from build123d import *

# Parameters (mm, degrees)
F1_DEPTH = 38.1
F2_R     = 5.08
F4_D     = 3.175


with BuildPart() as f1:
    # F0 (on Top) → F1 (new body)
    with BuildSketch(Plane.XY):
        with BuildLine():
            Line((32.319215, -2.299103), (32.319215, 1.700897))
            Line((32.319215, 1.700897), (36.015589, 1.700897))
            ThreePointArc((36.015589, 1.700897), (9.819215, 24.200897), (-16.377159, 1.700897))
            Line((-16.377159, 1.700897), (-12.680785, 1.700897))
            Line((-12.680785, 1.700897), (-12.680785, -2.299103))
            ThreePointArc((-12.680785, -2.299103), (9.819215, 20.200897), (32.319215, -2.299103))
        make_face()
        with BuildLine():
            Line((36.015589, 1.700897), (32.319215, 1.700897))
            Line((32.319215, 1.700897), (32.319215, -2.299103))
            Line((32.319215, -2.299103), (36.319215, -2.299103))
            ThreePointArc((36.319215, -2.299103), (36.2432, -0.293349), (36.015589, 1.700897))
        make_face()
        with BuildLine():
            Line((70.419215, 1.700897), (36.015589, 1.700897))
            ThreePointArc((36.015589, 1.700897), (36.2432, -0.293349), (36.319215, -2.299103))
            Line((36.319215, -2.299103), (70.419215, -2.299103))
            Line((70.419215, -2.299103), (70.419215, 1.700897))
        make_face()
        with BuildLine():
            Line((-12.680785, 1.700897), (-16.377159, 1.700897))
            ThreePointArc((-16.377159, 1.700897), (-16.604769, -0.293349), (-16.680785, -2.299103))
            Line((-16.680785, -2.299103), (-12.680785, -2.299103))
            Line((-12.680785, -2.299103), (-12.680785, 1.700897))
        make_face()
        with BuildLine():
            ThreePointArc((-16.680785, -2.299103), (-16.604769, -0.293349), (-16.377159, 1.700897))
            Line((-16.377159, 1.700897), (-50.780785, 1.700897))
            Line((-50.780785, 1.700897), (-50.780785, -2.299103))
            Line((-50.780785, -2.299103), (-16.680785, -2.299103))
        make_face()
    extrude(amount=F1_DEPTH)

    # F2
    f2_edges = [f1.edges().sort_by_distance(p)[0] for p in [
        (70.419215, -0.299103, 38.1),
        (70.419215, -0.299103, 0),
        (32.319215, -2.299103, 19.05),
        (-12.680785, -2.299103, 19.05),
        (-50.780785, -0.299103, 38.1),
        (-50.780785, -0.299103, 0),
        (-16.377159, 1.700897, 19.05),
        (36.015589, 1.700897, 19.05),
    ]]
    fillet(f2_edges, radius=F2_R)

    # F4 (through all)
    with Locations(Plane(origin=(0, 1.700897, 0), x_dir=(-1, 0, 0), z_dir=(0, 1, 0))):
        with Locations((-58.892906, 25.4), (-58.892906, 12.7), (38.062844, 12.7), (38.062844, 25.4)):
            Hole(F4_D / 2)


solid = f1.part
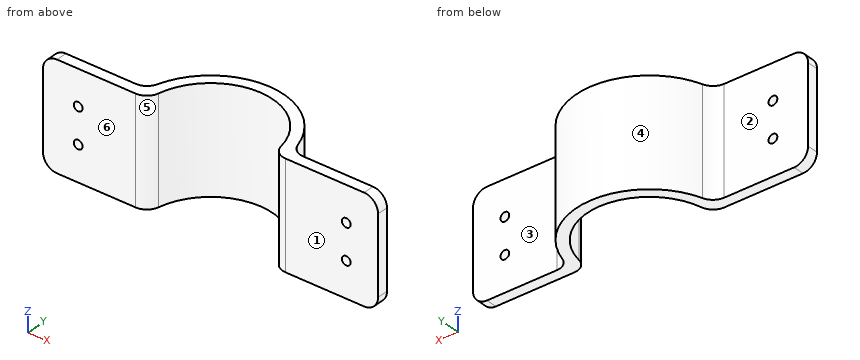
For this review, take the finished solid that the model builds, in its own axes (mm). Face numbers are marked on the shaded views. A direction names the side the tool comes from. Give positions to 0.01 mm unless a question says otherwise; leave off trailing zeros. Loops run counter-clockwise (first coordinate to the right, second up) from the corner with the lowest first, then second, coordinate; pieces in that order, holes last. Notation, with made-up numbers: M -2,39 L 51,39 A22 ccw 51,45 Z; hole C 22,85.5 d11. An arc over 180 degrees is marked long. Answer as a JSON object with one key per item and string values. Group by question number.
Q1. Add section B-B on z = 21. Give the boundary of the cut face in (x, y).
Q2. For probe 1 along Y at (x, z) = (41.5, 8.5); probe 2 along X at (y, z) = (16.5, 22.5); probe 3 along X at (y, z) = (15.5, 31), list the stretches that pass through material, from the lowest coordinate up. Write a range as [from, to].
Q3. Add section D-D on x = 19. Give the boundary of the cut face in (y, z).
Q4. Add section A-A on z = 12.7. Give the boundary of the cut face in (x, y).
Q5. Add section C-C on y = 11. Give the boundary of the cut face in (x, z).
Q6. Mouldability with a two-part tool opening along X and no side actions: class the marked faces 4, 5 and 6 as +X half, -X half, draft (parallel to the pull), parting line (faces both ways), or undercut.
Q7. Tool access review of the marked faces 1, 2 and 3: name each direction out of +Z, -Z, +X, -X, +Y, -Y from which nothing blocks a thin tool from reaching the whole face with its end or side.
Q8. Insertion check: P1, Ø15, axis at x = -40.5, z = 19, coming from the +Y side; P2, Ø12, axis at x = 39, y = 8, coming from the +Z side; P3, Ø8, axis at y = 11.5, z = 22.5, coming from the +X side; P4, Ø12, axis at y = 19.5, z = 16.5, coming from the +X side. Each pin has a flat end and moves straight along its axis. Give the tip position at first contact, or say it passes through.
Checked values:
{
 "1": {"outline": "M -50.78,-2.3 L -17.29,-2.3 A5.08 ccw -12.3,1.85 A22.5 cw 31.93,1.85 A5.08 ccw 36.93,-2.3 L 70.42,-2.3 L 70.42,1.7 L 40.07,1.7 A5.08 cw 35.2,5.32 A26.5 ccw -15.56,5.32 A5.08 cw -20.43,1.7 L -50.78,1.7 Z"},
 "2": {"probe 1": "[-2.3, 1.7]", "probe 2": "[-8.86, -2.54], [22.18, 28.5]", "probe 3": "[-9.81, -3.94], [23.58, 29.45]"},
 "3": {"outline": "M 18.24,0 L 22.56,0 L 22.56,38.1 L 18.24,38.1 Z"},
 "4": {"outline": "M -50.78,-2.3 L -39.65,-2.3 L -39.65,1.7 L -50.78,1.7 Z; M -36.48,-2.3 L -17.29,-2.3 A5.08 ccw -12.3,1.85 A22.5 cw 31.93,1.85 A5.08 ccw 36.93,-2.3 L 57.31,-2.3 L 57.31,1.7 L 40.07,1.7 A5.08 cw 35.2,5.32 A26.5 ccw -15.56,5.32 A5.08 cw -20.43,1.7 L -36.48,1.7 Z; M 60.48,-2.3 L 70.42,-2.3 L 70.42,1.7 L 60.48,1.7 Z"},
 "5": {"outline": "M -13.1,0 L -8.33,0 L -8.33,38.1 L -13.1,38.1 Z; M 27.97,0 L 32.74,0 L 32.74,38.1 L 27.97,38.1 Z"},
 "6": {"face 4": "parting line", "face 5": "undercut", "face 6": "draft"},
 "7": {"face 1": "+Z, -Z, +X, -X, -Y", "face 2": "+Z, -Z, -X, +Y", "face 3": "+Z, -Z, +X, +Y"},
 "8": {"P1": "y = 1.7", "P2": "z = 38.1", "P3": "x = 34.44", "P4": "x = 31.09"}
}
